Autodesk Inventor part; units mm, degrees
ref_plane "YZ Plane" through (0, 0, 0) normal (1, 0, 0) x (0, 1, 0)
ref_plane "XZ Plane" through (0, 0, 0) normal (0, 1, 0) x (-1, 0, 0)
ref_plane "XY Plane" through (0, 0, 0) normal (0, 0, 1) x (1, 0, 0)
sketch "Sketch1" plane through (0, 0, 0) normal (0, 1, 0) x (-1, 0, 0)
  line L0 (121.4597, 127.3409) -> (-56.3403, 127.3409)
  line L1 (-56.3403, 127.3409) -> (-56.3403, -126.6591)
  line L2 (-56.3403, -126.6591) -> (121.4597, -126.6591)
  line L3 (121.4597, -126.6591) -> (121.4597, 127.3409)
  point P0 (0, 0)
  dimension "d0" = 254
  dimension "d1" = 177.8
sketch "Sketch2" plane through (0, 0, 0) normal (0, 1, 0) x (-1, 0, 0)
  point P0 (0, 0)
extrude "Extrusion1" add sketch "Sketch1" along normal blind 8.89
sketch "Sketch3" plane through (0, 8.89, 0) normal (0, 1, 0) x (1, 0, 0)
  line L0 (30.9403, -114.6409) -> (30.9403, -108.2909)
  line L1 (-121.4597, -127.3409) -> (56.3403, -127.3409)
  line L2 (56.3403, -127.3409) -> (56.3403, 126.6591)
  line L3 (30.9403, -108.2909) -> (-96.0597, -108.2909)
  line L4 (-96.0597, -108.2909) -> (-96.0597, -114.6409)
  line L5 (-96.0597, -114.6409) -> (30.9403, -114.6409)
  line L6 (-121.4597, 126.6591) -> (-121.4597, -127.3409)
  line L7 (-96.0597, -108.2909) -> (-89.7097, -108.2909)
  line L8 (-89.7097, -108.2909) -> (-89.7097, -63.8409)
  line L9 (-89.7097, -63.8409) -> (-96.0597, -63.8409)
  line L10 (-96.0597, -63.8409) -> (-96.0597, -108.2909)
  line L11 (-96.0597, -63.8409) -> (30.9403, -63.8409)
  line L12 (30.9403, -63.8409) -> (30.9403, -70.1909)
  line L13 (30.9403, -70.1909) -> (-96.0597, -70.1909)
  line L14 (-96.0597, -70.1909) -> (-96.0597, -63.8409)
  line L15 (-35.7347, -114.6409) -> (-29.3847, -114.6409)
  line L16 (-29.3847, -114.6409) -> (-29.3847, -63.8409)
  line L17 (-29.3847, -63.8409) -> (-35.7347, -63.8409)
  line L18 (-35.7347, -63.8409) -> (-35.7347, -114.6409)
  point P0 (0, 0)
  dimension "d4" = 6.35
  dimension "d5" = 12.7
  dimension "d6" = 25.4
  dimension "d7" = 25.4
  dimension "d8" = 6.35
  dimension "d10" = 127
  dimension "d11" = 6.35
  dimension "d12" = 50.8
  dimension "d13" = 6.35
  dimension "d14" = 60.325
  dimension "d15" = 60.325
sketch "Sketch4" plane through (0, 8.89, 0) normal (0, 1, 0) x (1, 0, 0)
  point P0 (0, 0)
extrude "Extrusion2" cut sketch "Sketch3" against normal blind 5.08 contours L5 L16 L3 L0 | L5 L18 L3 L16 | L3 L18 L13 L16 | L5 L4 L3 L18 | L16 L11 L12 L13 | L13 L18 L11 L16 | L3 L10 L13 L8 | L13 L8 L11 L18 | L13 L10 L9 L8
sketch "Sketch5" plane through (0, 8.89, 0) normal (0, 1, 0) x (1, 0, 0)
  line L0 (-96.0597, -4.1509) -> (30.9403, -4.1509)
  line L1 (30.9403, -4.1509) -> (30.9403, -10.5009)
  line L2 (30.9403, -10.5009) -> (-96.0597, -10.5009)
  line L3 (-96.0597, -10.5009) -> (-96.0597, -4.1509)
  line L4 (-96.0597, -63.8409) -> (30.9403, -63.8409)
  line L5 (-121.4597, 126.6591) -> (-121.4597, -127.3409)
  circle A0 centre (4.1687, -32.0909) radius 20.4377
  circle A1 centre (4.1687, -32.0909) radius 26.7877
  line L6 (56.3403, -127.3409) -> (56.3403, 126.6591)
  point P0 (0, 0)
  dimension "d18" = 53.34
  dimension "d19" = 6.35
  dimension "d20" = 127
  dimension "d21" = 25.4
  dimension "d22" = 6.35
  dimension "d23" = 21.59
  dimension "d24" = 100.2284
  dimension "d25" = 52.1716
sketch "Sketch6" plane through (0, 8.89, 0) normal (0, 1, 0) x (1, 0, 0)
  point P0 (0, 0)
extrude "Extrusion3" cut sketch "Sketch5" against normal blind 5.08
sketch "Sketch7" plane through (0, 8.89, 0) normal (0, 1, 0) x (1, 0, 0)
  line L0 (30.9403, 55.5391) -> (-32.5597, 55.5391)
  line L1 (-32.5597, 55.5391) -> (-32.5597, 48.0334)
  line L2 (-32.5597, 48.0334) -> (30.9403, 48.0334)
  line L3 (30.9403, 48.0334) -> (30.9403, 55.5391)
  line L4 (56.3403, -127.3409) -> (56.3403, 126.6591)
  line L5 (30.9403, -4.1509) -> (30.9403, -10.5009)
  circle A0 centre (4.1687, 27.5991) radius 20.4343
  circle A1 centre (4.1687, 27.5991) radius 26.7843
  line L6 (-96.0597, -4.1509) -> (30.9403, -4.1509)
  line L7 (-96.0597, -63.8409) -> (30.9403, -63.8409)
  arc A2 (-11.6885, -10.5009) -> (20.0259, -10.5009) centre (4.1687, -32.0909) ccw
  point P0 (0, 0)
  dimension "d31" = 25.4
  dimension "d35" = 31.75
  dimension "d37" = 27.94
  dimension "d39" = 27.94
  dimension "d40" = 63.5
  dimension "d42" = 25.4
  dimension "d43" = 26.7716
  dimension "d44" = 26.7716
  dimension "d45" = 31.75
  dimension "d46" = 6.35
sketch "Sketch9" plane through (0, 8.89, 0) normal (0, 1, 0) x (1, 0, 0)
  point P0 (0, 0)
extrude "Extrusion4" cut sketch "Sketch7" against normal blind 5.08 contours A1 L2 | L2 A1
sketch "Sketch12" plane through (0, 8.89, 0) normal (0, 1, 0) x (1, 0, 0)
  point P0 (0, 0)
sketch "Sketch13" plane through (0, 8.89, 0) normal (0, 1, 0) x (1, 0, 0)
  line L0 (30.9403, 48.4271) -> (-24.9397, 48.4271)
  line L1 (-24.9397, 48.4271) -> (-24.9397, 54.7771)
  line L2 (-24.9397, 54.7771) -> (30.9403, 54.7771)
  line L3 (30.9403, 54.7771) -> (30.9403, 48.4271)
  line L4 (56.3403, -127.3409) -> (56.3403, 126.6591)
  line L5 (-96.0597, -4.1509) -> (30.9403, -4.1509)
  point P0 (0, 0)
  dimension "d53" = 6.35
  dimension "d54" = 25.4
  dimension "d55" = 55.88
  dimension "d56" = 52.578
extrude "Extrusion5" cut sketch "Sketch13" against normal blind 5.08
sketch "Sketch15" plane through (0, 8.89, 0) normal (0, 1, 0) x (1, 0, 0)
  point P0 (0, 0)
sketch "Sketch16" plane through (0, 8.89, 0) normal (0, 1, 0) x (1, 0, 0)
  point P0 (0, 0)
sketch "Sketch14" plane through (0, 8.89, 0) normal (0, 1, 0) x (1, 0, 0)
  line L0 (30.9403, 61.1271) -> (-23.4198, 61.1271)
  line L1 (-23.4198, 61.1271) -> (-23.4198, 67.4771)
  line L2 (-23.4198, 67.4771) -> (30.9403, 67.4771)
  line L3 (30.9403, 67.4771) -> (30.9403, 61.1271)
  line L4 (-24.9397, 54.7771) -> (30.9403, 54.7771)
  line L5 (-22.0163, 67.4771) -> (-15.6663, 67.4771)
  line L6 (-15.6663, 67.4771) -> (-15.6663, 82.7171)
  line L7 (-15.6663, 82.7171) -> (-22.0163, 82.7171)
  line L8 (-22.0163, 82.7171) -> (-22.0163, 67.4771)
  line L9 (-22.0163, 82.7171) -> (30.9403, 82.7171)
  line L10 (30.9403, 82.7171) -> (30.9403, 89.0671)
  line L11 (30.9403, 89.0671) -> (-22.0163, 89.0671)
  line L12 (-22.0163, 89.0671) -> (-22.0163, 82.7171)
  line L13 (-22.0163, 89.0671) -> (-15.6663, 89.0671)
  line L14 (-15.6663, 89.0671) -> (-15.6663, 104.3071)
  line L15 (-15.6663, 104.3071) -> (-22.0163, 104.3071)
  line L16 (-22.0163, 104.3071) -> (-22.0163, 89.0671)
  line L17 (-22.0163, 104.3071) -> (30.9403, 104.3071)
  line L18 (30.9403, 104.3071) -> (30.9403, 110.6571)
  line L19 (30.9403, 110.6571) -> (-22.0163, 110.6571)
  line L20 (-22.0163, 110.6571) -> (-22.0163, 104.3071)
  point P0 (0, 0)
  dimension "d59" = 6.35
  dimension "d60" = 6.35
  dimension "d61" = 6.35
  dimension "d62" = 15.24
  dimension "d63" = 6.35
  dimension "d64" = 15.24
  dimension "d65" = 6.35
  dimension "d66" = 6.35
extrude "Extrusion6" cut sketch "Sketch14" against normal blind 5.08
sketch "Sketch19" plane through (0, 3.81, 0) normal (0, 1, 0) x (1, 0, 0)
  point P0 (0, 0)
sketch "Sketch21" plane through (0, 8.89, 0) normal (0, 1, 0) x (1, 0, 0)
  circle A0 centre (-116.3797, -122.2609) radius 3.175
  line L0 (-121.4597, 126.6591) -> (-121.4597, -127.3409)
  line L1 (-121.4597, -127.3409) -> (56.3403, -127.3409)
  point P0 (0, 0)
  dimension "d69" = 6.35
  dimension "d70" = 5.08
  dimension "d71" = 5.08
sketch "Sketch22" plane through (0, 8.89, 0) normal (0, 1, 0) x (1, 0, 0)
  circle A0 centre (51.2603, -122.2609) radius 3.175
  line L0 (56.3403, -127.3409) -> (56.3403, 126.6591)
  line L1 (-121.4597, -127.3409) -> (56.3403, -127.3409)
  circle A1 centre (-116.3797, 121.5791) radius 3.175
  line L2 (56.3403, 126.6591) -> (-121.4597, 126.6591)
  line L3 (-121.4597, 126.6591) -> (-121.4597, -127.3409)
  circle A2 centre (51.2603, 121.5791) radius 3.175
  point P0 (0, 0)
  dimension "d72" = 6.35
  dimension "d73" = 5.08
  dimension "d74" = 5.08
  dimension "d75" = 6.35
  dimension "d76" = 5.08
  dimension "d77" = 5.08
  dimension "d78" = 6.35
  dimension "d79" = 5.08
  dimension "d80" = 5.08
extrude "Extrusion7" cut sketch "Sketch22" against normal blind 25.4 contours A0 | A1 | A2
extrude "Extrusion8" cut sketch "Sketch21" against normal blind 25.4
equation "\"BendRadius\" = Thickness"
equation "\"BendReliefWidth\" = Thickness"
equation "\"BendReliefDepth\" = 0.5 * Thickness"
equation "\"CornerReliefSize\" = 4 * Thickness"
equation "\"MinimumRemnant\" = 2 * Thickness"
equation "\"TransitionRadius\" = BendRadius"
equation "\"JacobiRadiusSize\" = Thickness"
equation "\"GapSize\" = Thickness"
properties part number "Adam Name Plate" material "Aluminum"
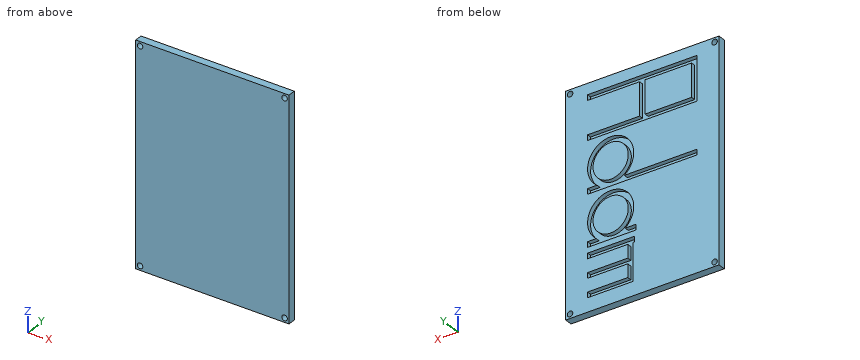
Source: CAD feature listing. Evaluate the final solid. Frame: model axes, mm. Round coordinates to 2 decimals unless told otherwise and drop trailing zeros. Write each loop counter-clockwise with the first axis right and the second up, starting at its lowest first coordinate (ties: lowest second). Pieces come first, ordered by that corner, then holes. Notation, with made-up numbers: M -9,-18.5 L 26,-18.5 A25 ccw 26,14.5 Z; hole C 47.5,-24.5 d11. An arc over 180 degrees is marked long. Answer as a JSON object with one key per item and string values. Group by question number.
(1) Section query A-A on z = 80.5. Output: boundary loops of the cut face in (x, y).
(2) Section query B-B on y = 5.5. State how many separate pieces and enclosed holes the cut face has, then the cut area to 3 significant figures.
(3) Ray query, line 1 (X direction, y = 7.5, z = 107.5); line 2 (Z direction, x = -34, y = 6.5); line 3 (X direction, y = 5.75, z = -72). Return the intervals inside material, ascending. Write a range as [from, to].
(4) Section query D-D on z = -71. Output: boundary loops of the cut face in (x, y).
Computed values:
{
 "1": {"outline": "M -121.46,0 L 56.34,0 L 56.34,8.89 L -29.38,8.89 L -29.38,3.81 L -35.73,3.81 L -35.73,8.89 L -89.71,8.89 L -89.71,3.81 L -96.06,3.81 L -96.06,8.89 L -121.46,8.89 Z"},
 "2": {"separate pieces": "4", "enclosed holes": "8", "area": "38,900 mm^2"},
 "3": {"line 1": "[-121.46, -96.06], [-89.71, -35.73], [-29.38, 56.34]", "line 2": "[-126.66, 4.15], [10.5, 63.84], [114.64, 127.34]", "line 3": "[-121.46, -22.02], [-15.67, 56.34]"},
 "4": {"outline": "M -121.46,0 L 56.34,0 L 56.34,8.89 L -15.67,8.89 L -15.67,3.81 L -22.02,3.81 L -22.02,8.89 L -121.46,8.89 Z"}
}
